from build123d import *

# Parameters (mm, degrees)
F1_DEPTH = 25.4
F2_R     = 25.43243
F3_DEPTH = 50.8
F4_R     = 12.7
F5_DEPTH = 177.8
F7_DEPTH = 203.2


with BuildPart() as f1:
    # F0 (on Top) → F1 (new body)
    with BuildSketch(Plane.XY):
        with BuildLine():
            Line((62.257019, 27.917736), (-52.042981, 27.917736))
            Line((-52.042981, 27.917736), (-52.042981, 27.772728))
            ThreePointArc((-52.042981, 27.772728), (-77.40406, 2.411649), (-52.042981, -22.94943))
            Line((-52.042981, -22.94943), (-52.042981, -23.094439))
            Line((-52.042981, -23.094439), (62.257019, -23.094439))
            Line((62.257019, -23.094439), (62.257019, -22.788397))
            ThreePointArc((62.257019, -22.788397), (87.457065, 2.411649), (62.257019, 27.611695))
            Line((62.257019, 27.611695), (62.257019, 27.917736))
        make_face()
    extrude(amount=F1_DEPTH)

    # F2 (on face) → F3 (join)
    with BuildSketch(Plane.XY.offset(25.4)):
        with Locations((-52.042981, 2.411649)):
            Circle(F2_R)
    extrude(amount=F3_DEPTH)

    # F4 (on face) → F5 (cut)
    with BuildSketch(Plane.XY.offset(76.2)):
        with Locations((-52.042981, 2.411649)):
            Circle(F4_R)
    extrude(amount=-F5_DEPTH, mode=Mode.SUBTRACT)

    # F6 (on face) → F7 (cut)
    with BuildSketch(Plane.XY.offset(25.4)):
        with BuildLine():
            Line((0, 18.215184), (0.714671, 18.198568))
            ThreePointArc((0.714671, 18.198568), (0.357432, 18.211029), (0, 18.215184))
        make_face()
        with BuildLine():
            Line((51.425615, 17.019568), (0.714671, 18.198568))
            Line((0.714671, 18.198568), (0, 18.215184))
            ThreePointArc((0, 18.215184), (-15.376876, 2.655535), (0.363372, -12.536422))
            Line((0.363372, -12.536422), (50.766153, -11.345099))
            ThreePointArc((50.766153, -11.345099), (65.278218, 2.507503), (51.425615, 17.019568))
        make_face()
    extrude(amount=-F7_DEPTH, mode=Mode.SUBTRACT)


solid = f1.part
Read the model definition and answer for the solid it produces. Units are mm, in the model's axes. A direction names the side the tool comes from. Coordinates: 2 decimals unless noted, no trailing zeros. Order: outer loops, then holes, each group sorted by start corner. A loop starts at its lowest first (then second) coordinate and runs counter-clockwise, first axis right, second up. Notation, with made-up numbers: M 83.25,-16 L 127.25,-16 A23 ccw 127.25,21 Z; hole C -17,73 d8. An arc over 180 degrees is marked long. Put each result on its own line as item: value. Start each with the question number.
Item 1: The mould has two halves that part along Y. Classify faces 1 (the face through (-15.377, 2.996, 12.878)), 2 (the face through (6, 27.918, 13)), 3 (the face through (32, -14, 25.4)): +Y half, -Y half, draft (parallel to the pull), parting line (faces both ways), or undercut.
Item 2: For faces 4 (the face through (65.268, 2.196, 12.878)), 5 (the face through (87.45, 1.86, 12.52)), 6 (the face through (-27.8, 10.1, 50.4)), determine the directions among +Z, -Z, +X, -X, +Y, -Y from which every point of the face is accessible in a straight line to the end or side of a thin tool.
Item 3: Section D-D, the plane z = 40 is taken. Determine the outline of the cut face in (x, y), plus the area to 3 significant figures.
Item 4: Consider probe 1 along X at (y, z) = (3.5, 4); probe 2 along Y at (x, z) = (-55.5, 27); probe 3 along X at (y, z) = (-4, 67.5). Determine where each line is inside the solid, lowest interval first. Write a range as [from, to].
Item 5: Section B-B, the plane y = 5.5 is taken. Determine the outline of the cut face in (x, z).
Item 6: Given pin 1 Ø12.5 at (x, y) = (-63, 11) entering from -Z; pin 2 Ø12 at (x, z) = (-51, 52) entering from -Y; pin 3 Ø2 at (y, z) = (0, 57) entering from -X; pin 4 Ø1 at (y, z) = (-12, 63.5) entering from -X, each flat-ended and moving along its own axis, determine where each tip first touches the part or whether it passes through.
Item 7: Section A-A, the plane x = -50.5 is taken. Determine the outline of the cut face in (y, z).
Item 8: Section C-C, the plane x = 13 is taken. Determine the outline of the cut face in (y, z), plus the area to 3 significant figures.
Computed:
1. face 1: undercut
1. face 2: +Y half
1. face 3: draft
2. face 4: +Z, -Z
2. face 5: +Z, -Z, +X
2. face 6: +Z
3. outline: C -52.04,2.41 d50.86; hole C -52.04,2.41 d25.4
3. area: 1,530 mm2
4. probe 1: x = [-77.38, -64.7], [-39.39, -15.36], [65.27, 87.43]
4. probe 2: y = [-22.78, -9.81], [14.63, 27.61]
4. probe 3: x = [-76.65, -63.01], [-41.08, -27.43]
5. outline: M -77.29,25.4 L -77.22,25.4 L -77.22,0 L -64.36,0 L -64.36,76.2 L -77.29,76.2 Z; M -39.72,0 L -15.15,0 L -15.15,25.4 L -26.8,25.4 L -26.8,76.2 L -39.72,76.2 Z; M 65.03,0 L 87.27,0 L 87.27,25.4 L 65.03,25.4 Z
6. pin 1: stops at z = 0
6. pin 2: stops at y = -23.02
6. pin 3: stops at x = -77.44
6. pin 4: stops at x = -73.33
7. outline: M -23.09,0 L -10.19,0 L -10.19,76.2 L -22.97,76.2 L -22.97,25.4 L -23.09,25.4 Z; M 15.02,0 L 27.92,0 L 27.92,25.4 L 27.8,25.4 L 27.8,76.2 L 15.02,76.2 Z
8. outline: M -23.09,0 L -12.24,0 L -12.24,25.4 L -23.09,25.4 Z; M 17.91,0 L 27.92,0 L 27.92,25.4 L 17.91,25.4 Z
8. area: 530 mm2
